Input: part model. Units: mm. Frame: model coordinates. Round coordinates to 2 decimals unless told otherwise and drop trailing zeros. Loops run counter-clockwise (first coordinate to the right, second up) from the corner with the lowest first, then second, coordinate; pieces in that order, holes last.
1) Ray query, line 1 along Y through (x, z) = (42.5, 0.9); line 2 along X through (y, z) = (46, 1.35); line 3 along Y through (x, z) = (67, 1.35). Return the intervals inside material, ascending.
2) Section D-D, the plane y = 45.5. Return loops of the section in (x, z).
3) Draft query along X for faces 1 (the face through (53.68, 59.24, 1.48)), 2 (the face through (48.027, 38.478, 1.479)), 3 (the face through (61.67, 53.91, 1.48)), 4 (the face through (53.59, 64.49, 1.48)). Return one class per face: pulls with the +X half, pulls with the -X half, needs draft (parallel to the pull), parting line crosses it, or undercut.
4) Section C-C, the plane x = 61.5. Return loops of the section in (y, z).
5) Section B-B, the plane z = 0.6. Return loops of the section in (x, y), and give its area (3 significant figures).
6) First-contact query: pin 1 (2 mm diameter, centred on x = 42.38, y = 15.73, fed in from -Z); pin 2 (1.5 mm diameter, centred on x = 44.5, z = 0.5, fed in from -Y). Flat tips, straight axial feed; report the tip coordinate or a pass-through.
7) Section A-A, the plane y = 15. Return loops of the section in (x, z).
from build123d import *

# Parameters (mm, degrees)
MODEL_R             = 1.300000002
MODEL_R_2           = 1.500000003
BOSS_EXTRUDE1_DEPTH = 3


with BuildPart() as part:
    # Model → Boss-Extrude1 (new body)
    with BuildSketch(Plane.XY):
        with BuildLine():
            ThreePointArc((57.913301974, 61.156066436), (53.502068591, 64.480518249), (49.975907149, 60.228795621))
            ThreePointArc((49.975907149, 60.228795621), (47.94925686, 38.176029403), (39.030226452, 17.905787524))
            ThreePointArc((39.030226452, 17.905787524), (40.582105252, 12.156647321), (46.129664865, 14.321254263))
            ThreePointArc((46.129664865, 14.321254263), (55.685249441, 30.675009463), (70.137725469, 42.917576284))
            ThreePointArc((70.137725469, 42.917576284), (72.036216679, 47.098079429), (68.754469063, 50.309155261))
            ThreePointArc((68.754469063, 50.309155261), (61.589228346, 53.988877576), (57.913301974, 61.156066436))
        make_face()
        with Locations((42.384943632, 15.727344886)):
            Circle(MODEL_R, mode=Mode.SUBTRACT)
        with Locations((53.966045378, 60.508142659)):
            Circle(MODEL_R, mode=Mode.SUBTRACT)
        with Locations((68.104570202, 46.36236227)):
            Circle(MODEL_R_2, mode=Mode.SUBTRACT)
    extrude(amount=BOSS_EXTRUDE1_DEPTH)


solid = part.part
Final values:
1. line 1: y = 11.73 to 14.43, 17.02 to 23.89
1. line 2: x = 49.5 to 66.65, 69.56 to 72.09
1. line 3: y = 40.92 to 45.35, 47.38 to 50.72
2. outline: (49.42, 0) - (66.88, 0) - (66.88, 3) - (49.42, 3) - close; (69.33, 0) - (72.01, 0) - (72.01, 3) - (69.33, 3) - close
3. face 1: undercut
3. face 2: pulls with the -X half
3. face 3: pulls with the +X half
3. face 4: parting line crosses it
4. outline: (36.64, 0) - (54.08, 0) - (54.08, 3) - (36.64, 3) - close
5. outline: (39.03, 17.91) arc R4 ccw (long way) to (46.13, 14.32) arc R56.11 cw to (70.14, 42.92) arc R4 ccw to (68.75, 50.31) arc R13.15 cw to (57.91, 61.16) arc R4 ccw to (49.98, 60.23) arc R68.89 cw to start; hole circle Ø2.6 at (42.38, 15.73); hole circle Ø2.6 at (53.97, 60.51); hole circle Ø3 at (68.1, 46.36)
5. area: 615 mm2
6. pin 1: passes through
6. pin 2: stops at y = 11.97
7. outline: (38.45, 0) - (41.31, 0) - (41.31, 3) - (38.45, 3) - close; (43.46, 0) - (46.39, 0) - (46.39, 3) - (43.46, 3) - close
